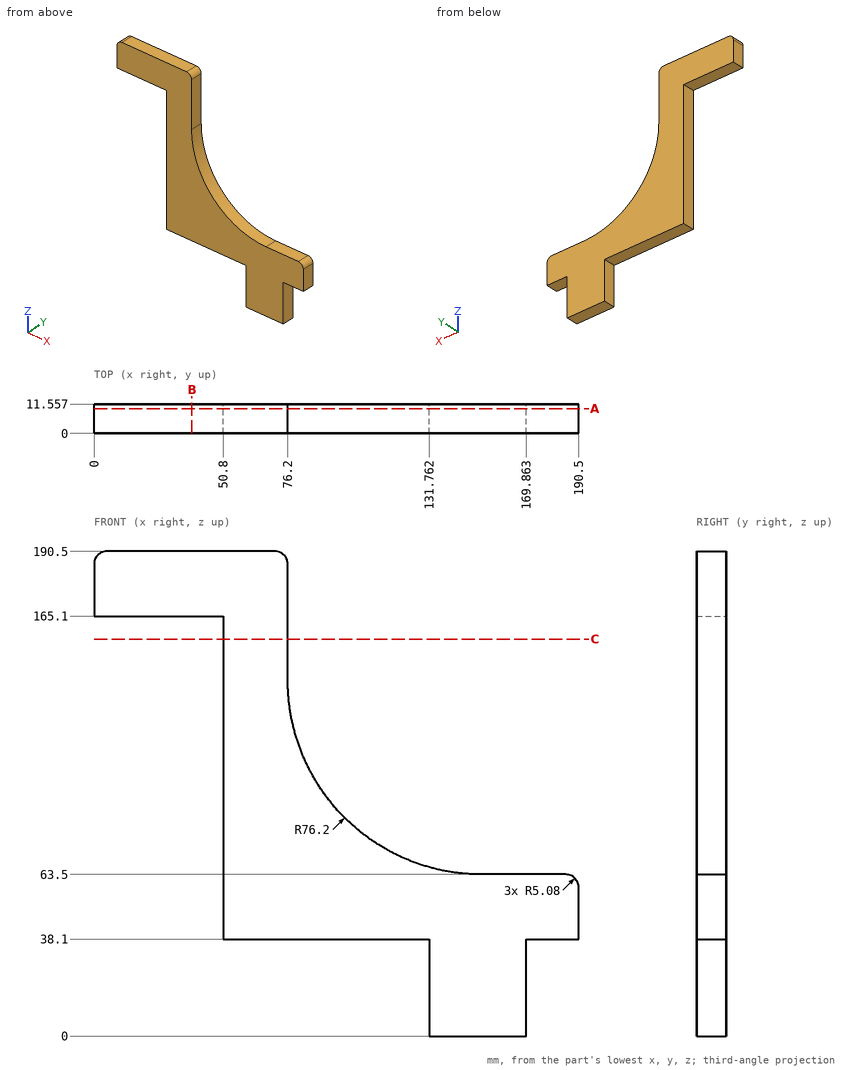
Input: dimensioned drawing with shaded views. Units: mm. Origin: part minimum x, y, z. Round coordinates to 2 decimals unless told otherwise and drop trailing zeros. Loops run counter-clockwise (first coordinate to the right, second up) from the corner with the lowest first, then second, coordinate; pieces in that order, holes last. Notation, with made-up numbers: (-22, 5.5) -> (-8, 5.5) arc R20 cw to (-8, 10.5) -> close; hole circle Ø9 at (30.25, 33.5). An arc over 180 degrees is marked (long way). Use one line per item in the form item = value. Start each with the question number.
1) First-contact query: P1, Ø6, axis at y = 3.5, z = 23.5, coming from the +X side; P2, Ø3.5, axis at y = 5.5, z = 160.5, coming from the +X side; P3, Ø3.5, axis at x = 182, y = 3, coming from the -Z side. Flat tips, straight axial feed; report the tip coordinate or a pass-through.
2) Section C-C on z = 156. Output: boundary loops of the cut face in (x, y).
3) Line query: L1, parallel to X at y = 11.25, z = 173; L2, parallel to X at y = 2.5, z = 38; L3, parallel to Z at x = 175.5, y = 3.75. Output: solid intervals per line, ascending.
4) Section B-B on x = 38.5. Output: boundary loops of the cut face in (y, z).
5) Section A-A on y = 9.75. Output: boundary loops of the cut face in (x, z), then the cut area to 3 significant figures.
Response:
q1.P1 = 169.86
q1.P2 = 76.2
q1.P3 = 38.1
q2.outline = (50.8, 0) -> (76.2, 0) -> (76.2, 11.56) -> (50.8, 11.56) -> close
q3.L1 = 0 to 76.2
q3.L2 = 131.76 to 169.86
q3.L3 = 38.1 to 63.5
q4.outline = (0, 165.1) -> (11.56, 165.1) -> (11.56, 190.5) -> (0, 190.5) -> close
q5.outline = (0, 165.1) -> (50.8, 165.1) -> (50.8, 38.1) -> (131.76, 38.1) -> (131.76, 0) -> (169.86, 0) -> (169.86, 38.1) -> (190.5, 38.1) -> (190.5, 58.42) arc R5.08 ccw to (185.42, 63.5) -> (152.4, 63.5) arc R76.2 cw to (76.2, 139.7) -> (76.2, 185.42) arc R5.08 ccw to (71.12, 190.5) -> (5.08, 190.5) arc R5.08 ccw to (0, 185.42) -> close
q5.area = 10,700 mm^2
